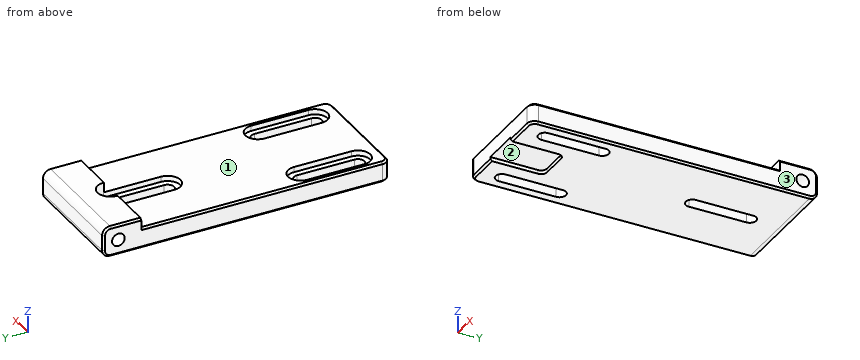
```python
from build123d import *

# Parameters (mm, degrees)
SKETCH1_W           = 30
SKETCH1_H           = 80
BOSS_EXTRUDE1_DEPTH = 8
CUT_EXTRUDE1_DEPTH  = 44.462627624
CUT_EXTRUDE2_DEPTH  = 4
CUT_EXTRUDE3_DEPTH  = 32
CUT_EXTRUDE4_DEPTH  = 4
SKETCH8_W           = 2.6
SKETCH8_H           = 70
CUT_EXTRUDE5_DEPTH  = 73
FILLET1_R           = 2
FILLET2_R           = 2
CHAMFER1_SIZE       = 0.5
CUT_EXTRUDE7_DEPTH  = 1
SKETCH10_W          = 41.633807812
SKETCH10_H          = 5
CUT_EXTRUDE8_DEPTH  = 10
FILLET3_R           = 2
CHAMFER2_SIZE       = 0.5


with BuildPart() as part:
    # Sketch1 → Boss-Extrude1 (new body)
    with BuildSketch(Plane.XY):
        Rectangle(SKETCH1_W, SKETCH1_H)
    extrude(amount=BOSS_EXTRUDE1_DEPTH)

    # Sketch3 → M4 Tapped Hole1 (revolve, cut)
    with BuildSketch(Plane(origin=(-15, 36, 4), x_dir=(0, 0, 1), z_dir=(0, 1, 0))):
        Polygon((0, 0), (0, 12.491420021), (1.65, 11.5), (1.65, 0), align=None)
    m4_tapped_hole1 = revolve(axis=Axis((-21.35, 36, 4), (1, 0, 0)), mode=Mode.SUBTRACT)

    # Mirror1: M4 Tapped Hole1 across plane
    add(m4_tapped_hole1.mirror(Plane.ZY), mode=Mode.SUBTRACT)

    # Sketch4 → Cut-Extrude1 (cut, through all)
    with BuildSketch(Plane(origin=(0, 0, 0), x_dir=(-1, 0, 0), z_dir=(0, 0, -1))):
        with BuildLine():
            Line((-8.8, -14), (-8.8, -29))
            ThreePointArc((-8.8, -29), (-10.5, -30.7), (-12.2, -29))
            Line((-12.2, -29), (-12.2, -14))
            ThreePointArc((-12.2, -14), (-10.5, -12.3), (-8.8, -14))
        make_face()
        with BuildLine():
            Line((8.8, -14), (8.8, -29))
            ThreePointArc((8.8, -29), (10.5, -30.7), (12.2, -29))
            Line((12.2, -29), (12.2, -14))
            ThreePointArc((12.2, -14), (10.5, -12.3), (8.8, -14))
        make_face()
    extrude(amount=-CUT_EXTRUDE1_DEPTH, mode=Mode.SUBTRACT)

    # Sketch5 → Cut-Extrude2 (cut)
    with BuildSketch(Plane.XY.offset(8)):
        with BuildLine():
            Line((-7.25, -14), (-7.25, -29))
            ThreePointArc((-7.25, -29), (-10.5, -32.25), (-13.75, -29))
            Line((-13.75, -29), (-13.75, -14))
            ThreePointArc((-13.75, -14), (-10.5, -10.75), (-7.25, -14))
        make_face()
        with BuildLine():
            Line((7.25, -14), (7.25, -29))
            ThreePointArc((7.25, -29), (10.5, -32.25), (13.75, -29))
            Line((13.75, -29), (13.75, -14))
            ThreePointArc((13.75, -14), (10.5, -10.75), (7.25, -14))
        make_face()
    extrude(amount=-CUT_EXTRUDE2_DEPTH, mode=Mode.SUBTRACT)

    # Sketch6 → Cut-Extrude3 (cut)
    with BuildSketch(Plane.XY.offset(8)):
        with BuildLine():
            Line((1.7, 30.14), (1.7, 15.14))
            ThreePointArc((1.7, 15.14), (0, 13.44), (-1.7, 15.14))
            Line((-1.7, 15.14), (-1.7, 30.14))
            ThreePointArc((-1.7, 30.14), (0, 31.84), (1.7, 30.14))
        make_face()
    extrude(amount=-CUT_EXTRUDE3_DEPTH, mode=Mode.SUBTRACT)

    # Sketch7 → Cut-Extrude4 (cut)
    with BuildSketch(Plane.XY.offset(8)):
        with BuildLine():
            Line((3.329829484, 30.14), (3.329829484, 15.14))
            ThreePointArc((3.329829484, 15.14), (0, 11.810170516), (-3.329829484, 15.14))
            Line((-3.329829484, 15.14), (-3.329829484, 30.14))
            ThreePointArc((-3.329829484, 30.14), (0, 33.469829484), (3.329829484, 30.14))
        make_face()
    extrude(amount=-CUT_EXTRUDE4_DEPTH, mode=Mode.SUBTRACT)

    # Sketch8 → Cut-Extrude5 (cut)
    with BuildSketch(Plane.ZY.offset(15)):
        with Locations((6.7, -5)):
            Rectangle(SKETCH8_W, SKETCH8_H)
    extrude(amount=-CUT_EXTRUDE5_DEPTH, mode=Mode.SUBTRACT)

    # Fillet1
    fillet1_edges = [part.edges().sort_by_distance(p)[0] for p in [
        (0, 40, 0),
        (0, 40, 8),
    ]]
    fillet(fillet1_edges, radius=FILLET1_R)

    # Fillet2
    fillet2_edges = [part.edges().sort_by_distance(p)[0] for p in [
        (15, -40, 2.7),
        (-15, -40, 2.7),
    ]]
    fillet(fillet2_edges, radius=FILLET2_R)

    # Chamfer1
    chamfer1_edges = [part.edges().sort_by_distance(p)[0] for p in [
        (15, 34, 8),
        (15, -4, 5.4),
        (-15, -4, 5.4),
        (-15, 34, 8),
        (-15, 40, 4),
        (-15, 0, 0),
        (-15, 39.414213562, 0.585786438),
        (-15, 39.414213562, 7.414213562),
        (15, 40, 4),
        (15, 39.414213562, 0.585786438),
        (15, 39.414213562, 7.414213562),
        (0, -40, 5.4),
        (0, -40, 0),
        (15, 0, 0),
        (14.414213562, -39.414213562, 0),
        (-14.414213562, -39.414213562, 0),
        (14.414213562, -39.414213562, 5.4),
        (-14.414213562, -39.414213562, 5.4),
    ]]
    chamfer(chamfer1_edges, length=CHAMFER1_SIZE)

    # Sketch9 → Cut-Extrude7 (cut)
    with BuildSketch(Plane(origin=(0, 0, 0), x_dir=(-1, 0, 0), z_dir=(0, 0, -1))):
        with BuildLine():
            Line((-5, -40), (5, -40))
            Line((5, -40), (5, -22.5))
            ThreePointArc((5, -22.5), (4.560660172, -21.439339828), (3.5, -21))
            Line((3.5, -21), (-3.5, -21))
            ThreePointArc((-3.5, -21), (-4.560660172, -21.439339828), (-5, -22.5))
            Line((-5, -22.5), (-5, -40))
        make_face()
    extrude(amount=-CUT_EXTRUDE7_DEPTH, mode=Mode.SUBTRACT)

    # Sketch10 → Cut-Extrude8 (cut)
    with BuildSketch(Plane.XY.offset(5.4)):
        with Locations((0.581549675, -37.5)):
            Rectangle(SKETCH10_W, SKETCH10_H)
    extrude(amount=-CUT_EXTRUDE8_DEPTH, mode=Mode.SUBTRACT)

    # Fillet3
    fillet3_edges = [part.edges().sort_by_distance(p)[0] for p in [
        (15, -35, 2.7),
        (-15, -35, 2.7),
    ]]
    fillet(fillet3_edges, radius=FILLET3_R)

    # Chamfer2
    chamfer2_edges = [part.edges().sort_by_distance(p)[0] for p in [
        (13.822875656, -34.822875656, 0),
        (9, -35, 0),
        (13.822875656, -34.822875656, 5.4),
        (-13.822875656, -34.822875656, 5.4),
        (0, -35, 5.4),
        (-13.822875656, -34.822875656, 0),
        (-9, -35, 0),
    ]]
    chamfer(chamfer2_edges, length=CHAMFER2_SIZE - 0.0001)  # a hair under: the kernel refuses the full size


solid = part.part
```
Geometry check sheet. Reference: the model listing, model coordinates, mm. Face numbers are marked on the shaded views. Give positions to 0.01 mm unless a question says otherwise; leave off trailing zeros. Loops run counter-clockwise (first coordinate to the right, second up) from the corner with the lowest first, then second, coordinate; pieces in that order, holes last. Notation, with made-up numbers: M 52.25,26.25 L 84.25,26.25 A16 cw 84.25,45.25 Z; hole C -29.5,46 d6. An arc over 180 degrees is marked long. Answer as CSV lines item,"result".
Item 1: Cross-section at D-D on y = 26. Record the cut outline in (x, z), and give its area (3 significant figures).
Values:
outline,"M -15,0.5 L -14.5,0 L -1.7,0 L -1.7,4 L -3.33,4 L -3.33,5.4 L -14.5,5.4 L -15,4.9 Z; M 1.7,0 L 14.5,0 L 15,0.5 L 15,4.9 L 14.5,5.4 L 3.33,5.4 L 3.33,4 L 1.7,4 Z"
area,"139 mm²"
Item 2: Cross-section at B-B on y = -18. Record the cut outline in (x, z).
Values:
outline,"M -15,0.5 L -14.5,0 L -12.2,0 L -12.2,4 L -13.75,4 L -13.75,5.4 L -14.5,5.4 L -15,4.9 Z; M -8.8,0 L 8.8,0 L 8.8,4 L 7.25,4 L 7.25,5.4 L -7.25,5.4 L -7.25,4 L -8.8,4 Z; M 12.2,0 L 14.5,0 L 15,0.5 L 15,4.9 L 14.5,5.4 L 13.75,5.4 L 13.75,4 L 12.2,4 Z"
Item 3: Release check for a two-part mould opening along Z. For the marked faces 1, 2 and 3 record: pulls with the +Z half, pulls with the -Z half, needs draft (parallel to the pull), parting line crosses it, or undercut.
Values:
face 1,"pulls with the +Z half"
face 2,"pulls with the -Z half"
face 3,"needs draft"
Item 4: Depth check by flat-ended pin: P1, Ø3, axis at y = 36, z = 4, coming from the +X side; P2, Ø1, axis at y = 17.5, z = 6, coming from the -X side (3 decimals); P3, Ø5, axis at x = -1.5, y = -25.5, coming from the -Z side; P4, Ø5.5, axis at x = -1, y = 17.5, coming from the +Z side. Enter the tip coordinate at first touch or a pass-through.
Values:
P1,"stops at x = 3.41"
P2,"passes through"
P3,"stops at z = 1"
P4,"stops at z = 5.4"
Item 5: Material ranges on line 1 (X direction, y = -21.5, z = 2); line 2 (Z direction, x = 12.25, y = 36); line 3 (Y direction, x = 7, z = 4), recorded low to high.
Values:
line 1,"x = -15 to -12.2, -8.8 to 8.8, 12.2 to 15"
line 2,"z = 0 to 2.35, 5.65 to 8"
line 3,"y = -35 to 34.35, 37.65 to 40"
Item 6: Cross-section at A-A on x = 10.5. Record the cut outline in (y, z), and give its area (3 significant figures).
Values:
outline,"M -35,0.5 L -34.5,0 L -30.7,0 L -30.7,4 L -32.25,4 L -32.25,5.4 L -34.5,5.4 L -35,4.9 Z; M -12.3,0 L 38,0 A2 ccw 40,2 L 40,6 A2 ccw 38,8 L 30,8 L 30,5.4 L -10.75,5.4 L -10.75,4 L -12.3,4 Z; hole C 36,4 d3.3"
area,"317 mm²"
Item 7: Cross-section at C-C on x = 0. Record the cut outline in (y, z).
Values:
outline,"M -35,1 L -21,1 L -21,0 L 13.44,0 L 13.44,4 L 11.81,4 L 11.81,5.4 L -34.5,5.4 L -35,4.9 Z; M 31.84,0 L 38,0 A2 ccw 40,2 L 40,6 A2 ccw 38,8 L 33.47,8 L 33.47,4 L 31.84,4 Z"
